from build123d import *

# Parameters (mm, degrees)
F0_W     = 25
F0_H     = 25
F1_DEPTH = 25
F2_W     = 12
F2_H     = 12
F3_DEPTH = 25
F4_W     = 12
F4_H     = 12
F5_DEPTH = 25
F6_W     = 12
F6_H     = 12
F7_DEPTH = 25


with BuildPart() as f1:
    # F0 (on Top) → F1 (new body)
    with BuildSketch(Plane.XY):
        with Locations((12.5, 12.5)):
            Rectangle(F0_W, F0_H)
    extrude(amount=F1_DEPTH)

    # F2 (on face) → F3 (cut)
    with BuildSketch(Plane.XY.offset(25)):
        with Locations((12.820027, 13.99222)):
            Rectangle(F2_W, F2_H)
    extrude(amount=-F3_DEPTH, mode=Mode.SUBTRACT)

    # F4 (on face) → F5 (cut)
    with BuildSketch(Plane(origin=(0, 25, 0), x_dir=(-1, 0, 0), z_dir=(0, 1, 0))):
        with Locations((-12.115697, 11.221583)):
            Rectangle(F4_W, F4_H)
    extrude(amount=-F5_DEPTH, mode=Mode.SUBTRACT)

    # F6 (on face) → F7 (cut)
    with BuildSketch(Plane.YZ.offset(25)):
        with Locations((13.033153, 14.205345)):
            Rectangle(F6_W, F6_H)
    extrude(amount=-F7_DEPTH, mode=Mode.SUBTRACT)


solid = f1.part
Geometry: final body of the model. Coordinates: model frame, mm. A direction names the side the tool comes from. Coordinates: 2 decimals unless noted, no trailing zeros. Order: outer loops, then holes, each group sorted by start corner. A loop starts at its lowest first (then second) coordinate and runs counter-clockwise, first axis right, second up.
(1) Material intervals for probe 1 along X at (y, z) = (3.5, 16.75); probe 2 along Y at (x, z) = (7, 4.25); probe 3 along X at (y, z) = (19.75, 16.25), sorted ascending.
(2) Section query C-C (x = 2.5). Return the cut outline in (y, z), plus the area to 3 significant figures.
(3) Section query D-D (y = 15.5). Return the cut outline in (x, z), plus the area to 3 significant figures.
(4) Access query for faces 5 (the face through (18.116, 23, 11)), 6 (the face through (22, 13, 8.205)), 7 (the face through (13, 7.992, 2)), 8 (the face through (12, 7, 0)). Directions: +Z, -Z, +X, -X, +Y, -Y. A direction counts if a zero-diameter tool reaches every point of the face in a straight line with its end or side. Return the directions, or none.
(5) Draft query along X for faces 1 (the face through (0, 12, 7)), 2 (the face through (12, 25, 18)), 3 (the face through (13, 19.992, 18)), 4 (the face through (25, 12, 7)). Return one class per face: pulls with the +X half, pulls with the -X half, needs draft (parallel to the pull), parting line crosses it, or undercut.
(6) Section query A-A (x = 17.75). Return the cut outline in (y, z), plus the area to 3 significant figures.
(7) Section query B-B (z = 18.25). Return the cut outline in (x, y), plus the area to 3 significant figures.
Solution:
1. probe 1: x = 0 to 6.12, 18.12 to 25
1. probe 2: y = 0 to 7.99, 19.99 to 25
1. probe 3: x = 0 to 6.12, 18.82 to 25
2. outline: (0, 0) - (25, 0) - (25, 25) - (0, 25) - close; hole (7.03, 8.21) - (19.03, 8.21) - (19.03, 20.21) - (7.03, 20.21) - close
2. area: 481 mm2
3. outline: (0, 0) - (6.82, 0) - (6.82, 5.22) - (6.12, 5.22) - (6.12, 8.21) - (0, 8.21) - close; (0, 20.21) - (6.82, 20.21) - (6.82, 25) - (0, 25) - close; (18.82, 0) - (25, 0) - (25, 8.21) - (18.82, 8.21) - close; (18.82, 20.21) - (25, 20.21) - (25, 25) - (18.82, 25) - close
3. area: 167 mm2
4. face 5: +Y, -Y
4. face 6: +X, -X
4. face 7: +Z, -Z
4. face 8: -Z, +X, -X, +Y, -Y
5. face 1: pulls with the -X half
5. face 2: needs draft
5. face 3: undercut
5. face 4: pulls with the +X half
6. outline: (0, 0) - (7.99, 0) - (7.99, 5.22) - (0, 5.22) - close; (0, 17.22) - (7.03, 17.22) - (7.03, 20.21) - (7.99, 20.21) - (7.99, 25) - (0, 25) - close; (19.99, 0) - (25, 0) - (25, 5.22) - (19.99, 5.22) - close; (19.99, 17.22) - (25, 17.22) - (25, 25) - (19.99, 25) - close
6. area: 166 mm2
7. outline: (0, 0) - (25, 0) - (25, 7.03) - (0, 7.03) - close; (0, 19.03) - (6.82, 19.03) - (6.82, 19.99) - (18.82, 19.99) - (18.82, 19.03) - (25, 19.03) - (25, 25) - (0, 25) - close
7. area: 313 mm2
